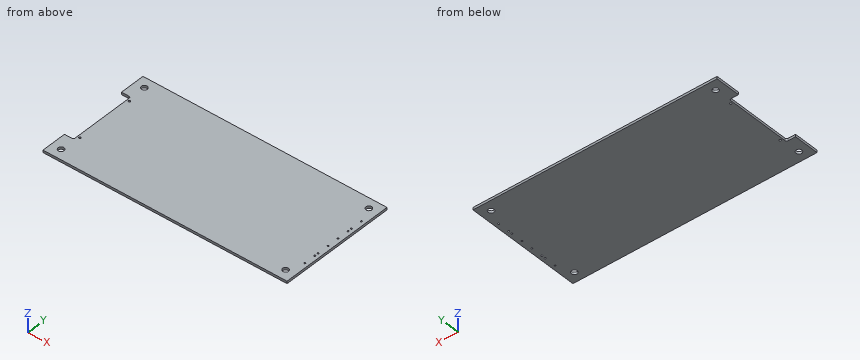
```python
from build123d import *

# Parameters (mm, degrees)
SKETCH1_W               = 158.75
SKETCH1_H               = 76.2
EXTRUDE1_DEPTH          = 1.5748
SKETCH2_R               = 1.905
CUT_EXTRUDE2_DEPTH      = 1.5748
SKETCH4_R               = 0.65
CUT_EXTRUDE3_DEPTH      = 1.5748
SKETCH5_R               = 0.508
TRANSCEIVER_HOLES_DEPTH = 2.54
LPATTERN1_COUNT         = 2
LPATTERN1_PITCH         = 25.4


with BuildPart() as part:
    # Sketch1 → Extrude1 (new body)
    with BuildSketch(Plane.XY):
        with Locations((79.375, -38.1)):
            Rectangle(SKETCH1_W, SKETCH1_H)
    extrude(amount=EXTRUDE1_DEPTH)

    # Sketch2 → Cut-Extrude2 (cut)
    with BuildSketch(Plane.XY.offset(1.5748)):
        with Locations((152.4, -6.35)):
            Circle(SKETCH2_R)
        with Locations((6.35, -6.35)):
            Circle(SKETCH2_R)
        with Locations((152.4, -69.85)):
            Circle(SKETCH2_R)
        with Locations((6.35, -69.85)):
            Circle(SKETCH2_R)
    extrude(amount=-CUT_EXTRUDE2_DEPTH, mode=Mode.SUBTRACT)

    # Sketch4 → Cut-Extrude3 (cut)
    with BuildSketch(Plane.XY.offset(1.5748)):
        with Locations((7.55, -19.234912)):
            Circle(SKETCH4_R)
        with Locations((7.55, -56.965088)):
            Circle(SKETCH4_R)
        with BuildLine():
            Line((0, -16.335006), (4.95, -16.335006))
            ThreePointArc((4.95, -16.335006), (5.657106781, -16.627899219), (5.95, -17.335006))
            Line((5.95, -17.335006), (5.95, -58.865006))
            ThreePointArc((5.95, -58.865006), (5.657106781, -59.572112781), (4.95, -59.865006))
            Line((4.95, -59.865006), (0, -59.865006))
            Line((0, -59.865006), (0, -16.335006))
        make_face()
    extrude(amount=-CUT_EXTRUDE3_DEPTH, mode=Mode.SUBTRACT)

    # Sketch5 → transceiver holes (cut)
    with BuildSketch(Plane.XY.offset(1.5748)):
        with Locations((156.21, -59.69)):
            Circle(SKETCH5_R)
        with Locations((156.21, -52.07)):
            Circle(SKETCH5_R)
        with Locations((156.21, -49.53)):
            Circle(SKETCH5_R)
        with Locations((156.21, -41.91)):
            Circle(SKETCH5_R)
    transceiver_holes = extrude(amount=-TRANSCEIVER_HOLES_DEPTH, mode=Mode.SUBTRACT)

    # LPattern1: transceiver holes ×2
    with Locations(*[(0, i * LPATTERN1_PITCH, 0) for i in range(1, LPATTERN1_COUNT)]):
        add(transceiver_holes, mode=Mode.SUBTRACT)


solid = part.part
```
Could you check a few things on this model? Use its own coordinates, in mm. Give positions to 0.01 mm unless a question says otherwise; leave off trailing zeros. Loops run counter-clockwise (first coordinate to the right, second up) from the corner with the lowest first, then second, coordinate; pieces in that order, holes last. Notation, with made-up numbers: (32, -2) - (57, -2) arc R24 cw to (57, 25) - close; hole circle Ø8 at (-23.75, -34). An arc over 180 degrees is marked (long way). Answer in a Markdown table with one row per item. Add a question column.
Q1. Please list where these lines run through material, in increasing order: L1, parallel to Y at x = 6.35, z = 0.3 (3 decimals); L2, parallel to X at y = -57, z = 1.3; L3, parallel to X at y = -34.29, z = 0.4. Write a range as from..to.
Q2. If we section it at A-A (y = -69.85): List the corners of the cut face in (x, z) for me (3 decimals).
Q3. If we section it at B-B (x = 152.4): List the corners of the cut face in (y, z) for me (3 decimals).
Q4. For pin 1 (1.2 mm diameter, centred on x = 7.55, y = -56.97, fed in from +Z), with a flat end and sliding along its axis, tell me the tip position at first contact or that it passes through.
Q5. If we section it at C-C (z = 0.95): State how many separate pieces and enclosed holes the cut face has, plus the area to 3 significant figures.
The answers:
| question | item | result |
|---|---|---|
| 1 | L1 | y = -76.2..-71.755, -67.945..-8.255, -4.445..0 |
| 1 | L2 | x = 5.95..6.9, 8.2..158.75 |
| 1 | L3 | x = 5.95..155.7, 156.72..158.75 |
| 2 | outline | (0, 0) - (4.445, 0) - (4.445, 1.575) - (0, 1.575) - close; (8.255, 0) - (150.495, 0) - (150.495, 1.575) - (8.255, 1.575) - close; (154.305, 0) - (158.75, 0) - (158.75, 1.575) - (154.305, 1.575) - close |
| 3 | outline | (-76.2, 0) - (-71.755, 0) - (-71.755, 1.575) - (-76.2, 1.575) - close; (-67.945, 0) - (-8.255, 0) - (-8.255, 1.575) - (-67.945, 1.575) - close; (-4.445, 0) - (0, 0) - (0, 1.575) - (-4.445, 1.575) - close |
| 4 | pin 1 | passes through |
| 5 | separate pieces | 1 |
| 5 | enclosed holes | 14 |
| 5 | area | 11,800 mm^2 |
